The model under review builds one solid part; all positions refer to its coordinate system, in mm. A direction names the side the tool comes from. Give positions to 0.01 mm unless a question says otherwise; leave off trailing zeros. Write each loop counter-clockwise with the first axis right and the second up, starting at its lowest first coordinate (ties: lowest second). Pieces come first, ordered by that corner, then holes. Notation, with made-up numbers: M -27.75,-28.75 L -17.75,-28.75 A16 cw -17.75,-23.75 Z; hole C 2.5,-3.75 d1. An arc over 180 degrees is marked long. Write item = value, one per line. Start each with the question number.
```python
from build123d import *

# Parameters (mm, degrees)
SKETCH2_R                       = 11.10996
BOSS_EXTRUDE1_DEPTH             = 4.7625
SKETCH3_W                       = 3.175
SKETCH3_H                       = 181.991160274
CUT_EXTRUDE1_DEPTH              = 0.396875
FILLET1_R                       = 0.79375
F_9_64_0_14063_DIAMETER_HOLE1_D = 3.572002
SKETCH8_W                       = 3.175
SKETCH8_H                       = 6.35
CUT_EXTRUDE2_DEPTH              = 163.951186269


with BuildPart() as part:
    # Sketch2 → Boss-Extrude1 (new body)
    with BuildSketch(Plane(origin=(0, 0, 0), x_dir=(0, 0, -1), z_dir=(1, 0, 0))):
        with BuildLine():
            Line((81.02619141, 88.258519733), (35.921024484, 114.3))
            ThreePointArc((35.921024484, 114.3), (0, 63.5), (-35.921024484, 114.3))
            Line((-35.921024484, 114.3), (-81.02619141, 88.258519733))
            ThreePointArc((-81.02619141, 88.258519733), (-54.99261314, 31.75), (-116.947215895, 26.041480267))
            Line((-116.947215895, 26.041480267), (-116.947215895, -26.041480267))
            ThreePointArc((-116.947215895, -26.041480267), (-54.99261314, -31.75), (-81.02619141, -88.258519733))
            Line((-81.02619141, -88.258519733), (-35.921024484, -114.3))
            ThreePointArc((-35.921024484, -114.3), (0, -63.5), (35.921024484, -114.3))
            Line((35.921024484, -114.3), (81.02619141, -88.258519733))
            ThreePointArc((81.02619141, -88.258519733), (54.99261314, -31.75), (116.947215895, -26.041480267))
            Line((116.947215895, -26.041480267), (116.947215895, 26.041480267))
            ThreePointArc((116.947215895, 26.041480267), (54.99261314, 31.75), (81.02619141, 88.258519733))
        make_face()
        with Locations(Location((0, 0, 0), (0, 0, 180))):
            Circle(SKETCH2_R, mode=Mode.SUBTRACT)
    extrude(amount=BOSS_EXTRUDE1_DEPTH)

    # Sketch3 → Cut-Extrude1 (cut)
    with BuildSketch(Plane.ZY):
        with Locations((0, 101.6)):
            Rectangle(SKETCH3_W, SKETCH3_H)
        Polygon((167.586415056, 94.92297474), (165.998915056, 97.672605397), (8.389946993, 6.67702526), (9.977446993, 3.927394603), align=None)
        Polygon((165.998915056, -97.672605397), (167.586415056, -94.92297474), (9.977446993, -3.927394603), (8.389946993, -6.67702526), align=None)
        with Locations((0, -101.6)):
            Rectangle(SKETCH3_W, SKETCH3_H)
        Polygon((-167.586415056, -94.92297474), (-165.998915056, -97.672605397), (-8.389946993, -6.67702526), (-9.977446993, -3.927394603), align=None)
        Polygon((-165.998915056, 97.672605397), (-167.586415056, 94.92297474), (-9.977446993, 3.927394603), (-8.389946993, 6.67702526), align=None)
    extrude(amount=-CUT_EXTRUDE1_DEPTH, mode=Mode.SUBTRACT)

    # Fillet1
    fillet1_edges = [part.edges().sort_by_distance(p)[0] for p in [
        (2.38125, 88.258519733, 81.02619141),
        (2.38125, 114.3, 35.921024484),
        (2.38125, 114.3, -35.921024484),
        (2.38125, 88.258519733, -81.02619141),
        (2.38125, 26.041480267, -116.947215895),
        (2.38125, -26.041480267, -116.947215895),
        (2.38125, -88.258519733, -81.02619141),
        (2.38125, -114.3, -35.921024484),
        (2.38125, -114.3, 35.921024484),
        (2.38125, -88.258519733, 81.02619141),
        (2.38125, -26.041480267, 116.947215895),
        (2.38125, 26.041480267, 116.947215895),
    ]]
    fillet(fillet1_edges, radius=FILLET1_R)

    # 9/64 (0.14063) Diameter Hole1 (through all)
    with Locations(Plane.ZY):
        with Locations((0, 25.4), (21.997045256, -12.7), (-21.997045256, -12.7)):
            Hole(F_9_64_0_14063_DIAMETER_HOLE1_D / 2)

    # Sketch8 → Cut-Extrude2 (cut, through all)
    with BuildSketch(Plane.ZY):
        with Locations((5.55625, 57.15)):
            Rectangle(SKETCH8_W, SKETCH8_H)
        with Locations((-5.55625, 57.15)):
            Rectangle(SKETCH8_W, SKETCH8_H)
        Polygon((44.759346169, 30.424538321), (43.171846169, 33.174168978), (48.671107483, 36.349168978), (50.258607483, 33.599538321), align=None)
        Polygon((54.227357483, 26.725461679), (55.814857483, 23.975831022), (50.315596169, 20.800831022), (48.728096169, 23.550461679), align=None)
        Polygon((48.728096169, -23.550461679), (50.315596169, -20.800831022), (55.814857483, -23.975831022), (54.227357483, -26.725461679), align=None)
        Polygon((50.258607483, -33.599538321), (48.671107483, -36.349168978), (43.171846169, -33.174168978), (44.759346169, -30.424538321), align=None)
        with Locations((5.55625, -57.15)):
            Rectangle(SKETCH8_W, SKETCH8_H)
        with Locations((-5.55625, -57.15)):
            Rectangle(SKETCH8_W, SKETCH8_H)
        Polygon((-44.759346169, -30.424538321), (-43.171846169, -33.174168978), (-48.671107483, -36.349168978), (-50.258607483, -33.599538321), align=None)
        Polygon((-54.227357483, -26.725461679), (-55.814857483, -23.975831022), (-50.315596169, -20.800831022), (-48.728096169, -23.550461679), align=None)
        Polygon((-48.728096169, 23.550461679), (-50.315596169, 20.800831022), (-55.814857483, 23.975831022), (-54.227357483, 26.725461679), align=None)
        Polygon((-50.258607483, 33.599538321), (-48.671107483, 36.349168978), (-43.171846169, 33.174168978), (-44.759346169, 30.424538321), align=None)
    extrude(amount=-CUT_EXTRUDE2_DEPTH, mode=Mode.SUBTRACT)


solid = part.part
```
Item 1: We need section B-B, the plane y = -50.8. Write out the cut boundary in (x, z), and give its area (3 significant figures).
Item 2: We need section C-C, the plane x = 3.85. Give the number of separate pieces and of enclosed holes in the cut face, and give its area (3 significant figures).
Item 3: For faces 5 (the flat face through (0.196, 20.191, 31.797)), 6 (the cylindrical face through (2.348, -63.513, 0.99)), list the 3-axis set-ups (+Z, -Z, +X, -X, +Y, -Y) from which the entire face can be reached by the end or side of a thin tool; tool diameter is ignored.
Item 4: We need section D-D, the plane z = 96. Write out the cut boundary in (x, y).
Item 5: To check wall thickness, follow probe 1 along Y at (x, z) = (1.8, 0); probe 2 along Y at (x, z) = (2.3, -73); probe 3 along Z at (x, y) = (1.7, -50.8). State the ranges of each line that lie inside material, in increasing order. Write a range as [from, to].
Item 6: We need section A-A, the plane y = 0. Write out the cut boundary in (x, z), and give its area (3 significant figures).
Item 7: The part is to be moulded in two halves that separate along Z. For faces 1 (the flat face through (0.196, -7.567, 16.282)), 2 (the flat face through (2.35, -101.45, -58.18)), 3 (the flat face through (0.397, -9, 15)), 4 (the flat face through (0, -59, -31)), say which applies: released by +Z, released by -Z, zero draft, split by the parting line, or undercut.
Item 8: Clearance check with flat-ended pins moving along their axes: P1, Ø1.6, axis at x = 3, z = -6.5, coming from the -Y side; P2, Ø1.6, axis at y = 21, z = 0, coming from the -X side; P3, Ø1.5, axis at x = 2, z = -49.5, coming from the -Y side; P4, Ø1.5, axis at x = 4, z = 37, coming from the -Y side. State where each tip first meets the part, or that it passes through.
Worked out:
q1.outline = M 0,-49.89 L 4.76,-49.89 L 4.76,49.89 L 0,49.89 L 0,1.59 L 0.4,1.59 L 0.4,-1.59 L 0,-1.59 Z
q1.area = 474 mm²
q2.separate_pieces = 1
q2.enclosed_holes = 16
q2.area = 22,900 mm²
q3.face_5 = -X
q3.face_6 = +X, -X
q4.outline = M 0,-13.55 L 4.76,-13.55 L 4.76,13.55 L 0,13.55 Z
q5.probe_1 = [-63.5, -11.11], [11.11, 23.61], [27.19, 63.5]
q5.probe_2 = [-92.89, -85.83], [-15.77, 15.77], [85.83, 92.89]
q5.probe_3 = [-49.89, 49.89]
q6.outline = M 0,-116.95 L 4.76,-116.95 L 4.76,-11.11 L 0,-11.11 Z; M 0,11.11 L 4.76,11.11 L 4.76,116.95 L 0,116.95 Z
q6.area = 1,010 mm²
q7.face_1 = undercut
q7.face_2 = released by -Z
q7.face_3 = undercut
q7.face_4 = zero draft
q8.P1 = -64.21
q8.P2 = 0.4
q8.P3 = -106.89
q8.P4 = -113.37
